Design review of the part built by this model. Coordinates are the model's own, in mm. Give positions to 0.01 mm unless a question says otherwise; leave off trailing zeros. Loops run counter-clockwise (first coordinate to the right, second up) from the corner with the lowest first, then second, coordinate; pieces in that order, holes last. Notation, with made-up numbers: M 57.25,15.25 L 101.25,15.25 A16 ccw 101.25,35.25 Z; hole C -32,19 d5. An arc over 180 degrees is marked long. Use one line per item in the form item = value. Start each with the question number.
from build123d import *

# Parameters (mm, degrees)
F0_W     = 255.2
F0_H     = 106.3
F0_R     = 3.25
F0_R_2   = 1.1
F0_R_3   = 7
F0_R_4   = 1.5
F1_DEPTH = 2.3


with BuildPart() as f1:
    # F0 (on Front) → F1 (new body)
    with BuildSketch(Plane.XZ):
        Rectangle(F0_W, F0_H)
        with Locations((-60, -18.15)):
            Circle(F0_R, mode=Mode.SUBTRACT)
        with Locations((-20, -18.15)):
            Circle(F0_R, mode=Mode.SUBTRACT)
        with Locations((-60, -12.95)):
            Circle(F0_R_2, mode=Mode.SUBTRACT)
        with Locations((-20, -12.95)):
            Circle(F0_R_2, mode=Mode.SUBTRACT)
        with Locations((20, -18.15)):
            Circle(F0_R, mode=Mode.SUBTRACT)
        with Locations((60, -18.15)):
            Circle(F0_R, mode=Mode.SUBTRACT)
        with Locations((20, -12.95)):
            Circle(F0_R_2, mode=Mode.SUBTRACT)
        with Locations((60, -12.95)):
            Circle(F0_R_2, mode=Mode.SUBTRACT)
        with Locations((-60, 16.85)):
            Circle(F0_R_3, mode=Mode.SUBTRACT)
        with Locations((-20, 16.85)):
            Circle(F0_R_3, mode=Mode.SUBTRACT)
        with Locations((-107.6, 33.15)):
            Circle(F0_R_4, mode=Mode.SUBTRACT)
        with Locations((20, 16.85)):
            Circle(F0_R_3, mode=Mode.SUBTRACT)
        with Locations((60, 16.85)):
            Circle(F0_R_3, mode=Mode.SUBTRACT)
    extrude(amount=-F1_DEPTH)


solid = f1.part
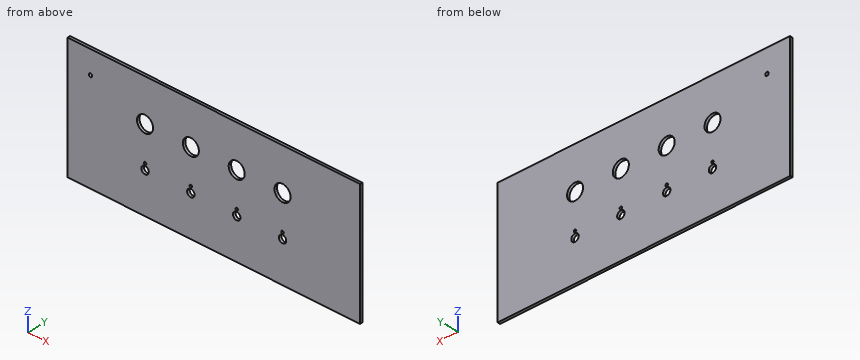
Q1. Take a section at B-B on y = 0.4. State how many separate pieces and enclosed holes the cut face has, plus the area to 3 significant figures.
Q2. Take a section at A-A on z = -18.15. Give the boundary of the cut face in (x, y), plus the area to 3 significant figures.
Q3. Wall thickness on probe 1 along Z at (x, y) = (-20, 1.75); probe 2 along Z at (x, y) = (-54, 0.4); probe 3 along X at (y, z) = (1.6, 19): over which ranges is each line inside the solid? List them lowest first.
Q4. Clearance check with flat-ended pins moving along their axes: pin 1 Ø7.5 at (x, z) = (-20, -18.15) entering from -Y; pin 2 Ø2 at (x, z) = (-20, -12.95) entering from +Y. State where each tip first meets the part, or that it passes through.
Q5. Take a section at C-C on z = 16.85. Give the boundary of the cut face in (x, y), plus the area to 3 significant figures.
Response values:
q1.separate_pieces = 1
q1.enclosed_holes = 13
q1.area = 26,400 mm^2
q2.outline = M -127.6,0 L -63.25,0 L -63.25,2.3 L -127.6,2.3 Z; M -56.75,0 L -23.25,0 L -23.25,2.3 L -56.75,2.3 Z; M -16.75,0 L 16.75,0 L 16.75,2.3 L -16.75,2.3 Z; M 23.25,0 L 56.75,0 L 56.75,2.3 L 23.25,2.3 Z; M 63.25,0 L 127.6,0 L 127.6,2.3 L 63.25,2.3 Z
q2.area = 527 mm^2
q3.probe_1 = -53.15 to -21.4, -14.9 to -14.05, -11.85 to 9.85, 23.85 to 53.15
q3.probe_2 = -53.15 to 13.24, 20.46 to 53.15
q3.probe_3 = -127.6 to -66.66, -53.34 to -26.66, -13.34 to 13.34, 26.66 to 53.34, 66.66 to 127.6
q4.pin_1 = 0
q4.pin_2 = through
q5.outline = M -127.6,0 L -67,0 L -67,2.3 L -127.6,2.3 Z; M -53,0 L -27,0 L -27,2.3 L -53,2.3 Z; M -13,0 L 13,0 L 13,2.3 L -13,2.3 Z; M 27,0 L 53,0 L 53,2.3 L 27,2.3 Z; M 67,0 L 127.6,0 L 127.6,2.3 L 67,2.3 Z
q5.area = 458 mm^2
